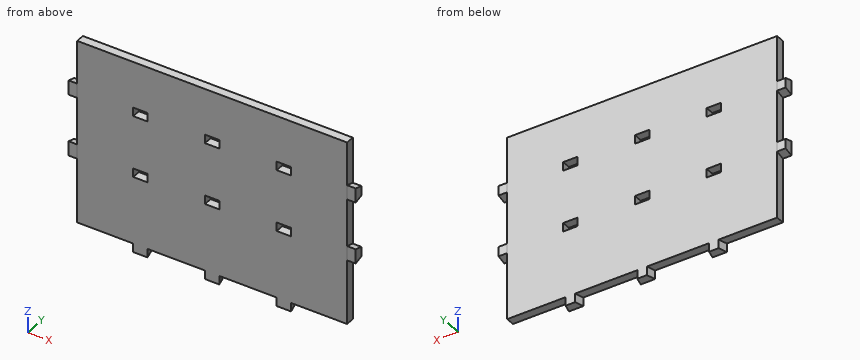
from build123d import *

# Parameters (mm, degrees)
F4_W      = 564.1347765923
F4_H      = 381.999976933
F5_DEPTH  = 18
F6_DEPTH  = 17.9999992251
F7_DEPTH  = 18.0000689332
F10_DEPTH = 17.8651544745
F12_DEPTH = 25


with BuildPart() as f5:
    # F4 (on plane+point) → F5 (new body)
    with BuildSketch(Plane.XZ.offset(-129.0130399809)):
        with Locations((-0.1316666603, 208.9999876916)):
            Rectangle(F4_W, F4_H)
    extrude(amount=F5_DEPTH)

    # F0 (on Top) → F6 (join, through all)
    with BuildSketch(Plane.XY):
        Polygon((149.935790569, 129.0130399809), (139.935790569, 129.0130399809), (134.935790569, 111.0130399809), (164.935790569, 111.0130399809), (159.935790569, 129.0130399809), align=None)
        Polygon((-0.064209431, 129.0130399809), (-10.064209431, 129.0130399809), (-15.064209431, 111.0130399809), (-0.064209431, 111.0130399809), (14.935790569, 111.0130399809), (9.935790569, 129.0130399809), align=None)
        Polygon((-150.064209431, 129.0130399809), (-160.064209431, 129.0130399809), (-165.064209431, 111.0130399809), (-135.064209431, 111.0130399809), (-140.064209431, 129.0130399809), align=None)
    extrude(amount=F6_DEPTH)

    # F3 (on plane+point) → F7 (join, through all)
    with BuildSketch(Plane.YZ.offset(299.935790569)):
        Polygon((111.0131509304, 152), (129.0131509304, 157), (129.0131509304, 177), (111.0131509304, 182), align=None)
        Polygon((129.0131509304, 295), (129.0131509304, 305), (111.0131509304, 310), (111.0131509304, 295), (111.0131509304, 280), (129.0131509304, 285), align=None)
    extrude(amount=-F7_DEPTH)

    # F9 (on offset) → F10 (join, through all)
    with BuildSketch(Plane.YZ.offset(-300.064209431)):
        Polygon((129.0131062269, 295), (129.0131062269, 305), (111.0131062269, 310), (111.0131062269, 295), (111.0131062269, 280), (129.0131062269, 285), align=None)
        Polygon((111.0131062269, 152), (129.0131062269, 157), (129.0131062269, 177), (111.0131062269, 182), align=None)
    extrude(amount=F10_DEPTH)

    # F11 (on plane+point) → F12 (cut)
    with BuildSketch(Plane.XZ.offset(-129.0130399809)):
        Polygon((164.9357974529, 167), (164.9357974529, 175.9999990463), (149.935790569, 175.9999990463), (134.9357962608, 175.9999990463), (134.9357962608, 167), (134.9357962608, 158.0000072718), (149.935790569, 158.0000072718), (164.9357974529, 158.0000072718), align=None)
        Polygon((149.935790569, 286.0000133514), (164.9357974529, 286.0000133514), (164.9357974529, 295), (164.9357974529, 303.9999902248), (149.935790569, 303.9999902248), (134.9357962608, 303.9999902248), (134.9357962608, 295), (134.9357962608, 286.0000133514), align=None)
        Polygon((14.9357905611, 167), (14.9357905611, 175.9999990463), (-15.0642096996, 175.9999990463), (-15.0642096996, 167), (-15.0642096996, 158.0000072718), (14.9357905611, 158.0000072718), align=None)
        Polygon((-15.0642096996, 286.0000133514), (14.9357905611, 286.0000133514), (14.9357905611, 295), (14.9357905611, 303.9999902248), (-15.0642096996, 303.9999902248), (-15.0642096996, 295), align=None)
        Polygon((-135.064214468, 167), (-135.064214468, 175.9999990463), (-165.0642156601, 175.9999990463), (-165.0642156601, 167), (-165.0642156601, 158.0000072718), (-135.064214468, 158.0000072718), align=None)
        Polygon((-165.0642156601, 286.0000133514), (-135.064214468, 286.0000133514), (-135.064214468, 295), (-135.064214468, 303.9999902248), (-165.0642156601, 303.9999902248), (-165.0642156601, 295), align=None)
    extrude(amount=F12_DEPTH, mode=Mode.SUBTRACT)


solid = f5.part
The listing builds one solid part. Answer for the finished solid, in the listing's coordinates (mm). Coordinates: 2 decimals unless noted, no trailing zeros. Write each loop counter-clockwise with the first axis right and the second up, starting at its lowest first coordinate (ties: lowest second). Pieces come first, ordered by that corner, then holes. Notation, with made-up numbers: M 42,-34 L 91,-34 A20 cw 91,-27 Z; hole C 31.25,-38.75 d9. An arc over 180 degrees is marked long. Put each result on its own line as item: value. Start each with the question number.
1. A cutting plane is placed at C-C on x = 49.5. Write down the section's boundary in (y, z), then the cut area to 3 significant figures.
2. A cutting plane is placed at A-A on x = 152. Write down the section's boundary in (y, z).
3. Flat-ended cylindrical pins translate along their axes: P1, Ø1.5, axis at y = 122.5, z = 327, coming from the +X side; P2, Ø2, axis at y = 125, z = 185, coming from the -X side; P3, Ø1.5, axis at x = -188, y = 126, coming from the -Z side. Find the tip coordinate at first contact, or state that the pin passes through.
4. A cutting plane is placed at B-B on z = 142. Write down the section's boundary in (x, y).
5. Consider line 1 (Z direction, x = 164, y = 119.25); line 2 (Z direction, x = -7, y = 121); line 3 (Z direction, x = -225.5, y = 122.75). Determine where each line is inside the solid, lowest interval first. Write a range as from..to.
6. A cutting plane is placed at D-D on y = 117.75. Count the separate pieces of the cut face and the enclosed holes in it, then the cut area to 3 significant figures.
Resolved:
1. outline: M 111.01,18 L 129.01,18 L 129.01,400 L 111.01,400 Z
1. area: 6,880 mm2
2. outline: M 111.01,0 L 129.01,0 L 129.01,158 L 111.01,158 Z; M 111.01,176 L 129.01,176 L 129.01,286 L 111.01,286 Z; M 111.01,304 L 129.01,304 L 129.01,400 L 111.01,400 Z
3. P1: stops at x = 281.94
3. P2: stops at x = -282.2
3. P3: stops at z = 18
4. outline: M -282.2,111.01 L 281.94,111.01 L 281.94,129.01 L -282.2,129.01 Z
5. line 1: z = 18..158, 176..286, 304..400
5. line 2: z = 0..158, 176..286, 304..400
5. line 3: z = 18..400
6. separate pieces: 1
6. enclosed holes: 6
6. area: 216,000 mm2
